Could you check a few things on this drawing? It's one solid part, dimensions in mm from its lowest x, y, z. A direction names the side the tool comes from. Give positions to 0.01 mm unless a question says otherwise; leave off trailing zeros. Order: outer loops, then holes, each group sorted by start corner. A loop starts at its lowest first (then second) coordinate and runs counter-clockwise, first axis right, second up.
(1) On a 3-axis mill with a long thin cutter (end or side, diameter ignored), from which of +Z, -Z, +X, -X, +Y, -Y can I reach the whole of each face in a straight line? I mean the marked faces 4, 5, 6, 7 and 8. Say none if no direction works.
(2) Imagine slicing it at B-B, the plane y = 55. Write out the boundary of the cut face in (x, z).
(3) Imagine slicing it at C-C, the plane y = 10. Write out the boundary of the cut face in (x, z), then the cut area to 3 significant figures.
(4) Imagine slicing it at A-A, the plane y = 71. Write out the boundary of the cut face in (x, z).
(5) Imagine slicing it at D-D, the plane z = 16.5. Write out the boundary of the cut face in (x, y).
(6) Will these pins go through, and if not, where does the flat tip stop? pin 1 (10 mm diameter, centred on x = 43, z = 14.5, fed in from +Y); pin 2 (13.5 mm diameter, centred on y = 9.5, z = 7, fed in from -X); pin 3 (6 mm diameter, centred on x = 25.5, z = 15.5, fed in from -Y).
(7) If we mould it in two halves opening along X, with no side actions, what happens to the marked faces 1, 2 and 3? For each: released by +X, released by -X, zero draft, split by the parting line, or undercut.
(8) If I drill on probe 1 along Z at (x, y) = (1, 55); probe 2 along X at (y, z) = (37.5, 10.75); probe 3 along X at (y, z) = (16, 7), over which ranges is the centre line in solid material (lowest first)?
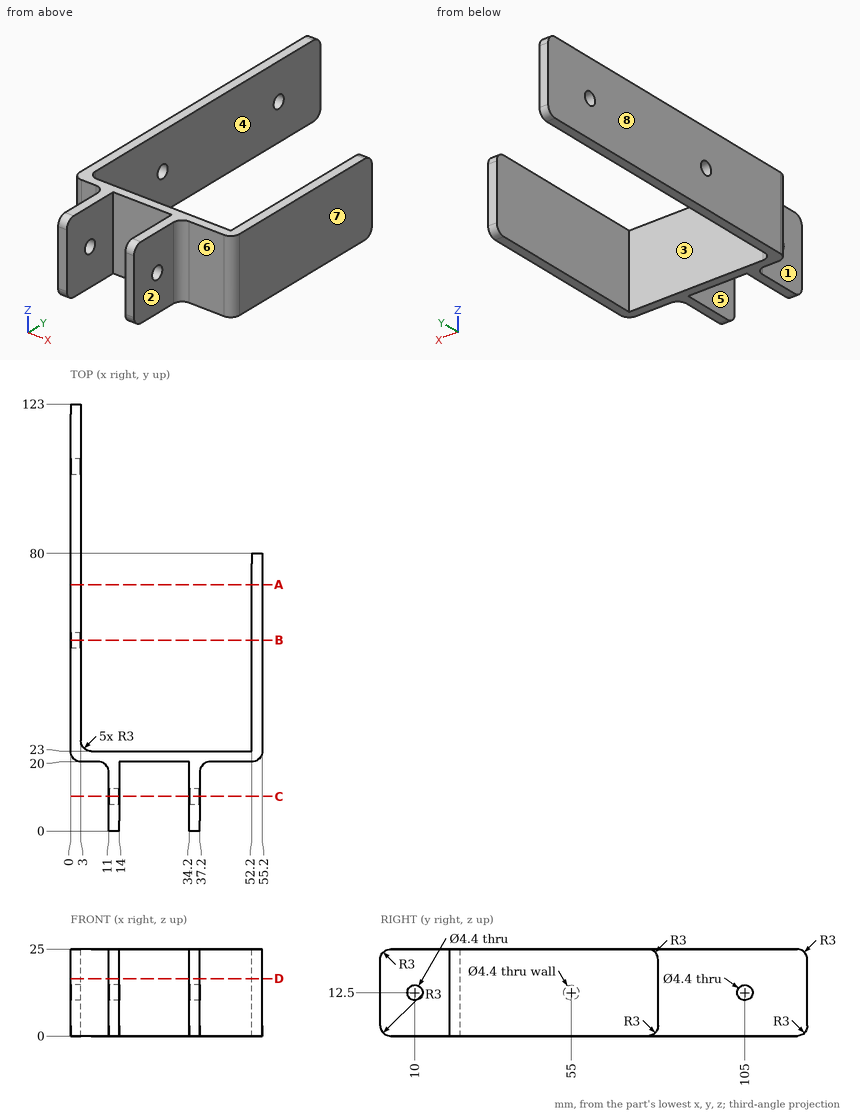
Answer block:
1. face 4: +Z, -Z, +Y
1. face 5: +Z, -Z, -Y
1. face 6: +Z, -Z, +X, -Y
1. face 7: +Z, -Z, +X, +Y, -Y
1. face 8: +Z, -Z, -X, +Y, -Y
2. outline: (0, 0) - (3, 0) - (3, 10.3) - (0, 10.3) - close; (0, 14.7) - (3, 14.7) - (3, 25) - (0, 25) - close; (52.2, 0) - (55.2, 0) - (55.2, 25) - (52.2, 25) - close
3. outline: (11, 0) - (14, 0) - (14, 10.3) - (11, 10.3) - close; (11, 14.7) - (14, 14.7) - (14, 25) - (11, 25) - close; (34.2, 0) - (37.2, 0) - (37.2, 10.3) - (34.2, 10.3) - close; (34.2, 14.7) - (37.2, 14.7) - (37.2, 25) - (34.2, 25) - close
3. area: 124 mm2
4. outline: (0, 0) - (3, 0) - (3, 25) - (0, 25) - close; (52.2, 0) - (55.2, 0) - (55.2, 25) - (52.2, 25) - close
5. outline: (0, 23) arc R3 ccw to (3, 20) - (8, 20) arc R3 cw to (11, 17) - (11, 0) - (14, 0) - (14, 20) - (34.2, 20) - (34.2, 0) - (37.2, 0) - (37.2, 17) arc R3 cw to (40.2, 20) - (52.2, 20) arc R3 ccw to (55.2, 23) - (55.2, 80) - (52.2, 80) - (52.2, 23) - (6, 23) arc R3 cw to (3, 26) - (3, 123) - (0, 123) - close
6. pin 1: stops at y = 23
6. pin 2: stops at x = 11
6. pin 3: stops at y = 20
7. face 1: released by -X
7. face 2: released by +X
7. face 3: undercut
8. probe 1: z = 0 to 10.3, 14.7 to 25
8. probe 2: x = 0 to 3, 52.2 to 55.2
8. probe 3: x = 11 to 14, 34.2 to 37.2
